Can you work these out from the model? Positions are in its coordinate system, mm. A direction names the side the tool comes from. Give positions to 0.01 mm unless a question says otherwise; leave off trailing zeros. Loops run counter-clockwise (first coordinate to the right, second up) from the corner with the lowest first, then second, coordinate; pieces in that order, holes last. Notation, with made-up numbers: (11.5, 63.5) - (30.5, 63.5) arc R21 cw to (30.5, 77.5) - close; hole circle Ø9 at (42, 87.25). An arc over 180 degrees is marked (long way). Answer as a JSON object with one key per item and string values. Group by question number.
Item 1: Will these pins go through, and if not, where does the flat tip stop? pin 1 (1.6 mm diameter, centred on y = 7.5, z = 2, fed in from -X); pin 2 (6 mm diameter, centred on x = 35, y = 9.5, fed in from +Z); pin 3 (4.5 mm diameter, centred on x = 47, z = 6.6, fed in from -Y).
Item 2: Suppose I cut it at D-D on x = 2. Write out the boundary of the cut face in (y, z).
Item 3: Which directions (+Z, -Z, +X, -X, +Y, -Y) give clear straight access to the entire face, cutting with the end or side of a thin tool? Please do faces 4 (the flat face through (30, 23, 10)), 5 (the flat face through (0, 11, 2)), 6 (the flat face through (33, 12, 3.2)).
Item 4: Please list where these lines run through material, in increasing order: L1, parallel to Z at x = 47, y = 23.15; L2, parallel to X at y = 11, z = 2.5; L3, parallel to Y at x = 3, z = 8.25.
Item 5: Suppose I cut it at B-B on z = 6.6. Write out the boundary of the cut face in (x, y), and give its area (3 significant figures).
Item 6: Suppose I cut it at C-C on y = 22.5. Write out the boundary of the cut face in (x, z), and give its area (3 significant figures).
Item 7: Thinking about a two-plate mould opening in X: for faces 1 (the flat face through (-5, 23, 5)), 2 (the cylindrical face through (13.98, 23.09, 7.54)), 3 (the flat face through (30, 21.612, 6)), which applies, pulls with the +X half, pulls with the -X half, needs draft (parallel to the pull), parting line crosses it, or undercut?
Item 8: Suppose I cut it at A-A on x = 47. Write out the boundary of the cut face in (y, z).
from build123d import *

# Parameters (mm, degrees)
BOSS_EXTRUDE1_DEPTH = 67
SKETCH2_W           = 72
SKETCH2_H           = 10
BOSS_EXTRUDE2_DEPTH = 3
SKETCH3_R           = 1.3890625
CUT_EXTRUDE1_DEPTH  = 3


with BuildPart() as part:
    # Sketch1 → Boss-Extrude1 (new body)
    with BuildSketch(Plane(origin=(0, 0, 0), x_dir=(0, 0, -1), z_dir=(1, 0, 0))):
        Polygon((0, 0), (-3.2, 2.112416059), (-3.2, 21.612416059), (0, 21.612416059), align=None)
    extrude(amount=BOSS_EXTRUDE1_DEPTH)

    # Sketch2 → Boss-Extrude2 (add)
    with BuildSketch(Plane(origin=(0, 21.612416059, 0), x_dir=(1, 0, 0), z_dir=(0, 1, 0))):
        with Locations((31, -5)):
            Rectangle(SKETCH2_W, SKETCH2_H)
    extrude(amount=BOSS_EXTRUDE2_DEPTH)

    # Sketch3 → Cut-Extrude1 (cut)
    with BuildSketch(Plane.XZ.offset(-21.612416059)):
        with Locations((47, 6.6)):
            Circle(SKETCH3_R)
        with Locations((15, 6.6)):
            Circle(SKETCH3_R)
    extrude(amount=-CUT_EXTRUDE1_DEPTH, mode=Mode.SUBTRACT)


solid = part.part
Worked out:
{
 "1": {"pin 1": "stops at x = 0", "pin 2": "stops at z = 3.2", "pin 3": "stops at y = 21.61"},
 "2": {"outline": "(0, 0) - (24.61, 0) - (24.61, 10) - (21.61, 10) - (21.61, 3.2) - (2.11, 3.2) - close"},
 "3": {"face 4": "+Z, +X, -X, +Y, -Y", "face 5": "+Z, -Z, -X, -Y", "face 6": "+Z, +X, -X, -Y"},
 "4": {"L1": "z = 0 to 5.21, 7.99 to 10", "L2": "x = 0 to 67", "L3": "y = 21.61 to 24.61"},
 "5": {"outline": "(-5, 21.61) - (13.61, 21.61) - (13.61, 24.61) - (-5, 24.61) - close; (16.39, 21.61) - (45.61, 21.61) - (45.61, 24.61) - (16.39, 24.61) - close; (48.39, 21.61) - (67, 21.61) - (67, 24.61) - (48.39, 24.61) - close", "area": "199 mm2"},
 "6": {"outline": "(-5, 0) - (67, 0) - (67, 10) - (-5, 10) - close; hole circle Ø2.78 at (15, 6.6); hole circle Ø2.78 at (47, 6.6)", "area": "708 mm2"},
 "7": {"face 1": "pulls with the -X half", "face 2": "undercut", "face 3": "needs draft"},
 "8": {"outline": "(0, 0) - (24.61, 0) - (24.61, 5.21) - (21.61, 5.21) - (21.61, 3.2) - (2.11, 3.2) - close; (21.61, 7.99) - (24.61, 7.99) - (24.61, 10) - (21.61, 10) - close"}
}
